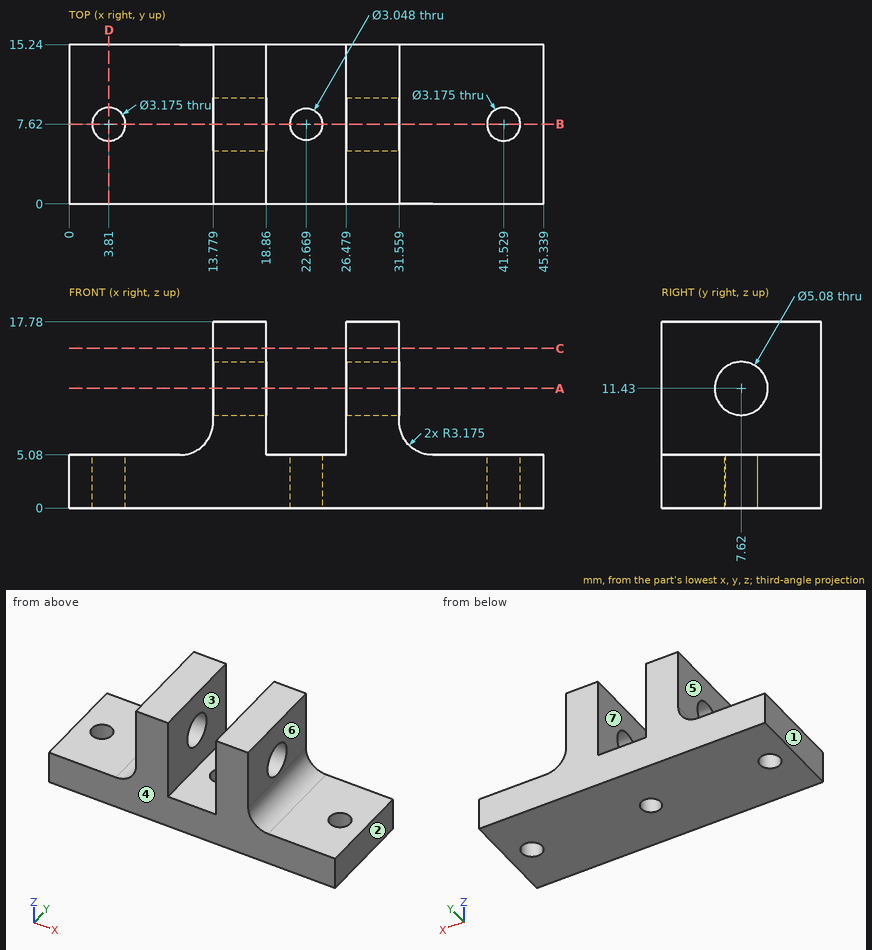
Geometry: see drawing. Coordinates: mm, zero at the bounding-box minimum. A direction names the side the tool comes from. Give positions to 0.01 mm unless a question says otherwise; leave off trailing zeros. Order: outer loops, then holes, each group sorted by start corner. A loop starts at its lowest first (then second) coordinate and runs counter-clockwise, first axis right, second up. Notation, with made-up numbers: (-15.5, -25.75) - (20.5, -25.75) arc R13 cw to (20.5, -16.75) - close; hole circle Ø10 at (62, 70.5). An arc over 180 degrees is marked (long way). Use CSV: the item, a comma, the result in double quotes.
1. Section query A-A (z = 11.43). Output: boundary loops of the cut face in (x, y).
Answers below:
outline,"(13.78, 0) - (18.86, 0) - (18.86, 5.08) - (13.78, 5.08) - close; (13.78, 10.16) - (18.86, 10.16) - (18.86, 15.24) - (13.78, 15.24) - close; (26.48, 0) - (31.56, 0) - (31.56, 5.08) - (26.48, 5.08) - close; (26.48, 10.16) - (31.56, 10.16) - (31.56, 15.24) - (26.48, 15.24) - close"
2. Access query for the marked faces 5, 6 and 7. Directions: +Z, -Z, +X, -X, +Y, -Y. A direction counts if a zero-diameter tool reaches every point of the face in a straight line with its end or side. Return the directions, or none.
Answers below:
face 5,"+Z, -X, +Y, -Y"
face 6,"+Z, +X, +Y, -Y"
face 7,"+Z, +Y, -Y"
3. Section query D-D (x = 3.81). Output: boundary loops of the cut face in (y, z).
Answers below:
outline,"(0, 0) - (6.03, 0) - (6.03, 5.08) - (0, 5.08) - close; (9.21, 0) - (15.24, 0) - (15.24, 5.08) - (9.21, 5.08) - close"
4. Mould query, pull axis X, two halves, no side actions, for the marked faces 1, 2, 3 and 4. Classes: +X half, -X half, draft (parallel to the pull), parting line (faces both ways), or undercut.
Answers below:
face 1,"-X half"
face 2,"+X half"
face 3,"undercut"
face 4,"draft"
5. Section query C-C (z = 15.25). Output: boundary loops of the cut face in (x, y), plus the area to 3 significant figures.
Answers below:
outline,"(13.78, 0) - (18.86, 0) - (18.86, 15.24) - (13.78, 15.24) - close; (26.48, 0) - (31.56, 0) - (31.56, 15.24) - (26.48, 15.24) - close"
area,"155 mm2"
6. Section query B-B (y = 7.62). Give the number of separate pieces and of enclosed holes in the cut face, plus the area to 3 significant figures.
Answers below:
separate pieces,"6"
enclosed holes,"0"
area,"264 mm2"
7. Contact query for flat-ended pins moving along their axis: pin 1 (3 mm diameter, centred on y = 7.5, z = 13.5, fed in from +X); pin 2 (4.5 mm diameter, centred on y = 7.62, z = 11.43, fed in from +X); pin 3 (5.5 mm diameter, centred on x = 39, y = 10, fed in from +Z); pin 4 (4 mm diameter, centred on y = 11, z = 9, fed in from -X). Output: stop coordinate, or through.
Answers below:
pin 1,"x = 31.56"
pin 2,"through"
pin 3,"z = 5.08"
pin 4,"x = 13.52"
8. Material intervals for line 1 along Y through (x, z) = (30.1, 11.43); line 2 along X through (y, z) = (5.25, 10.25); line 3 along Z through (x, y) = (5.5, 10.75), sorted ascending. Write a range as from..to.
Answers below:
line 1,"0..5.08, 10.16..15.24"
line 2,"13.78..18.86, 26.48..31.56"
line 3,"0..5.08"
